Drawing for the job (mm, zero at the part's lowest x, y, z). Round coordinates to 2 decimals unless told otherwise and drop trailing zeros. Loops run counter-clockwise (first coordinate to the right, second up) from the corner with the lowest first, then second, coordinate; pieces in that order, holes last. Notation, with made-up numbers: (-29.5, 23.5) - (3.5, 23.5) arc R17 ccw to (3.5, 44.5) - close; hole circle Ø3 at (36, -25). An arc over 180 degrees is marked (long way). Put each result on its own line as item: value.
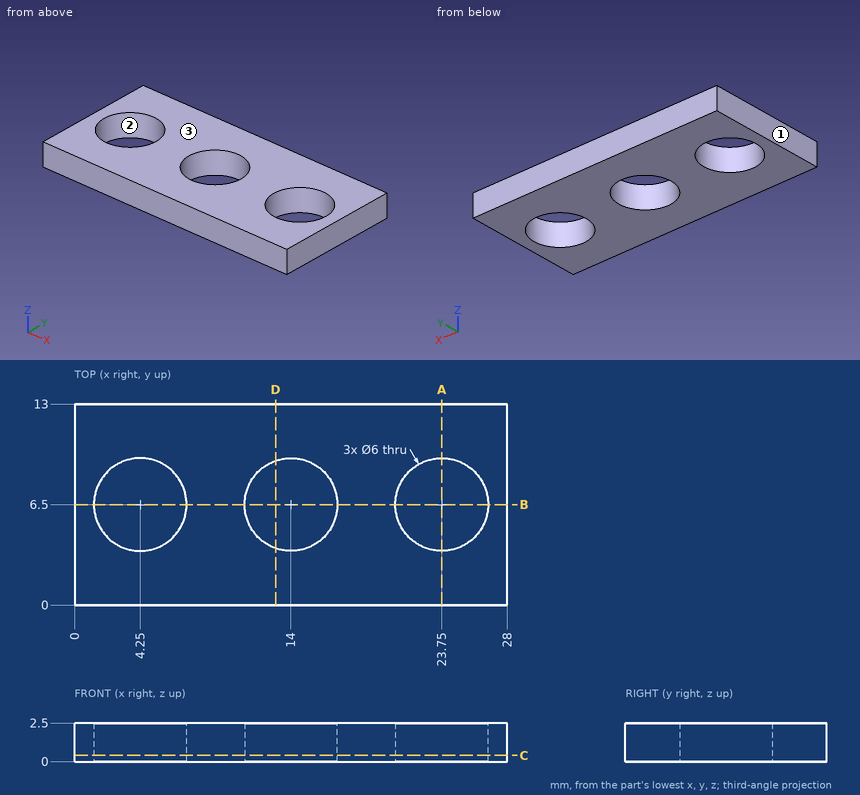
1. Probe line 1 along Y through (x, z) = (14, 0.9); line 2 along X through (y, z) = (5.25, 1.05); line 3 along Y through (x, z) = (5.5, 0.2). List the from-to ranges inside material, lowest first. Write a range as [from, to].
A:
line 1: y = [0, 3.5], [9.5, 13]
line 2: x = [0, 1.52], [6.98, 11.27], [16.73, 21.02], [26.48, 28]
line 3: y = [0, 3.77], [9.23, 13]
2. Band-saw the part on C-C (z = 0.4). List the corners of the cut face in (x, y), plus the area to 3 significant figures.
A:
outline: (0, 0) - (28, 0) - (28, 13) - (0, 13) - close; hole circle Ø6 at (4.25, 6.5); hole circle Ø6 at (14, 6.5); hole circle Ø6 at (23.75, 6.5)
area: 279 mm²
3. Band-saw the part on D-D (x = 13). List the corners of the cut face in (y, z).
A:
outline: (0, 0) - (3.67, 0) - (3.67, 2.5) - (0, 2.5) - close; (9.33, 0) - (13, 0) - (13, 2.5) - (9.33, 2.5) - close
4. Band-saw the part on B-B (y = 6.5). List the corners of the cut face in (x, z), plus the area to 3 significant figures.
A:
outline: (0, 0) - (1.25, 0) - (1.25, 2.5) - (0, 2.5) - close; (7.25, 0) - (11, 0) - (11, 2.5) - (7.25, 2.5) - close; (17, 0) - (20.75, 0) - (20.75, 2.5) - (17, 2.5) - close; (26.75, 0) - (28, 0) - (28, 2.5) - (26.75, 2.5) - close
area: 25.0 mm²
5. Two-plate mould, pull along X, no slides. Class the marked faces 1, 2 and 3: pulls with the +X half, pulls with the -X half, needs draft (parallel to the pull), parting line crosses it, or undercut.
A:
face 1: pulls with the -X half
face 2: undercut
face 3: needs draft
6. Band-saw the part on A-A (x = 23.75). List the corners of the cut face in (y, z), plus the area to 3 significant figures.
A:
outline: (0, 0) - (3.5, 0) - (3.5, 2.5) - (0, 2.5) - close; (9.5, 0) - (13, 0) - (13, 2.5) - (9.5, 2.5) - close
area: 17.5 mm²
